Autodesk Inventor part; units mm, degrees
ref_plane "YZ Plane" through (0, 0, 0) normal (1, 0, 0) x (0, 1, 0)
ref_plane "XZ Plane" through (0, 0, 0) normal (0, 1, 0) x (-1, 0, 0)
ref_plane "XY Plane" through (0, 0, 0) normal (0, 0, 1) x (1, 0, 0)
sketch "スケッチ1" plane through (0, 0, 0) normal (0, 1, 0) x (-1, 0, 0)
  line L0 (37.5, 1.5) -> (-37.5, 1.5)
  line L1 (-37.5, 1.5) -> (-37.5, -1.5)
  line L2 (-37.5, -1.5) -> (37.5, -1.5)
  line L3 (37.5, -1.5) -> (37.5, 1.5)
  line L4 (37.5, 1.5) -> (-37.5, -1.5) construction
  line L5 (-37.5, 1.5) -> (37.5, -1.5) construction
  line L6 (36.5, 3.5) -> (38.5, 3.5)
  line L7 (38.5, 3.5) -> (38.5, -3.5)
  line L8 (38.5, -3.5) -> (36.5, -3.5)
  line L9 (36.5, -3.5) -> (36.5, 3.5)
  line L10 (36.5, 3.5) -> (38.5, -3.5) construction
  line L11 (38.5, 3.5) -> (36.5, -3.5) construction
  line L12 (-36.5, 3.5) -> (-38.5, 3.5)
  line L13 (-38.5, 3.5) -> (-38.5, -3.5)
  line L14 (-38.5, -3.5) -> (-36.5, -3.5)
  line L15 (-36.5, -3.5) -> (-36.5, 3.5)
  line L16 (-36.5, 3.5) -> (-38.5, -3.5) construction
  line L17 (-38.5, 3.5) -> (-36.5, -3.5) construction
  point P0 (0, 0)
  point P1 (37.5, 0)
  point P2 (-37.5, 0)
  dimension "d0" = 75
  dimension "d1" = 3
  dimension "d2" = 2
  dimension "d3" = 7
  dimension "d4" = 2
  dimension "d5" = 7
extrude "押し出し1" add sketch "スケッチ1" along normal blind 78
sketch "スケッチ2" plane through (0, 78, 0) normal (0, 1, 0) x (1, 0, 0)
  line L0 (1.55, -1.5) -> (-1.55, -1.5)
  line L1 (-1.55, -1.5) -> (-1.55, 1.5)
  line L2 (-1.55, 1.5) -> (1.55, 1.5)
  line L3 (1.55, 1.5) -> (1.55, -1.5)
  line L4 (1.55, -1.5) -> (-1.55, 1.5) construction
  line L5 (-1.55, -1.5) -> (1.55, 1.5) construction
  point P0 (0, 0)
  dimension "d8" = 3.1
  dimension "d9" = 3
extrude "押し出し2" cut sketch "スケッチ2" against normal blind 39
fillet "フィレット1" radius 0.5 33 edges at (19.025, 78, -1.5) (19.025, 78, 1.5) (1.55, 78, 0) (1.55, 58.5, 1.5) (1.55, 58.5, -1.5) (-1.55, 58.5, -1.5) (0, 39, -1.5) (0, 39, 1.5) (-1.55, 58.5, 1.5) (-1.55, 78, 0) (-19.025, 78, 1.5) (-19.025, 78, -1.5) (36.5, 78, 2.5) (37.5, 78, 3.5) (38.5, 78, 0) (37.5, 78, -3.5) (36.5, 78, -2.5) (36.5, 39, -3.5) (38.5, 39, -3.5) (38.5, 39, 3.5) (36.5, 39, 3.5) (-36.5, 39, 3.5) (-37.5, 78, 3.5) (-36.5, 78, 2.5) (-38.5, 78, 0) (-36.5, 78, -2.5) (-37.5, 78, -3.5) (-36.5, 39, -3.5) (-38.5, 39, -3.5) (-38.5, 39, 3.5) (-38.5, 0, 0) (-37.5, 0, 3.5) (-36.5, 0, 2.5)
fillet "フィレット2" radius 0.5 20 edges at (-36.75, 0, 1.5) (0, 0, 1.5) (0, 0, -1.5) (-37, 0, -2.25) (-37, 0, 2.25) (-37.5, 0, 3) (36.6464, 0, 3.3536) (-38, 0, 0) (-37.5, 0, -3) (38.3536, 0, 3.3536) (38.3536, 0, -3.3536) (36.6462, 0, -3.3538) (-38.3536, 0.1464, 3) (-38.5, 0.5, 0) (-38.3536, 0.1464, -3) (37.5, 0, 3.5) (38.5, 0, 0) (37.4995, 0, -3.5) (36.5, 0, -2.2505) (36.5, 0, 2.25)
properties part number "partition"
Source: CAD feature listing. Evaluate the final solid. Frame: model axes, mm. A direction names the side the tool comes from. Coordinates: 2 decimals unless noted, no trailing zeros. Loops run counter-clockwise (first coordinate to the right, second up) from the corner with the lowest first, then second, coordinate; pieces in that order, holes last. Notation, with made-up numbers: (86, 73.25) -> (125, 73.25) arc R10 cw to (125, 87.25) -> close; hole circle Ø1 at (41, -39.75). An arc over 180 degrees is marked (long way). One line per item, written item: value. Start each with the question number.
Q1. Section query C-C, the plane y = 20. Return the cut outline in (x, z), and give its area (3 significant figures).
Q2. Section query B-B, the plane x = -8.5. Return the cut outline in (y, z), and give its area (3 significant figures).
Q3. Section query A-A, the plane y = 63. Return the cut outline in (x, z), and give its area (3 significant figures).
Q4. Mould query, pull axis X, two halves, no side actions, for faces 1 (the face through (21, 78, 0)), 2 (the face through (1, 38, -1.5)), 3 (the face through (38.5, 38, 0)). Classes: pulls with the +X half, pulls with the -X half, needs draft (parallel to the pull), parting line crosses it, or undercut.
Q5. Set-up query: faces 4 (the face through (1.55, 59, 0)), 5 (the face through (-1, 38, 1.5)), 6 (the face through (-38.5, 38, 0)). Return all of +Z, -Z, +X, -X, +Y, -Y with unobstructed straight access to the full face (end or side cutting, diameter ignored); none if empty.
Q6. Contact query for flat-ended pins moving along their axis: P1, Ø1, axis at x = -22, y = 16, coming from the -Z side; P2, Ø1, axis at x = -15, y = 27.5, coming from the +Z side; P3, Ø1, axis at x = -0.5, z = 0, coming from the +Y side. Output: stop coordinate, or through.
Q7. Line query: line 1 along X through (y, z) = (57.5, 0); line 2 along X through (y, z) = (47, -2.75); line 3 along Z through (x, y) = (-34, 20.5). Output: solid intervals per line, ascending.
Results:
1. outline: (-38.5, -3) arc R0.5 ccw to (-38, -3.5) -> (-37, -3.5) arc R0.5 ccw to (-36.5, -3) -> (-36.5, -1.5) -> (36.5, -1.5) -> (36.5, -3) arc R0.5 ccw to (37, -3.5) -> (38, -3.5) arc R0.5 ccw to (38.5, -3) -> (38.5, 3) arc R0.5 ccw to (38, 3.5) -> (37, 3.5) arc R0.5 ccw to (36.5, 3) -> (36.5, 1.5) -> (-36.5, 1.5) -> (-36.5, 3) arc R0.5 ccw to (-37, 3.5) -> (-38, 3.5) arc R0.5 ccw to (-38.5, 3) -> close
1. area: 247 mm^2
2. outline: (0, -1) arc R0.5 ccw to (0.5, -1.5) -> (77.5, -1.5) arc R0.5 ccw to (78, -1) -> (78, 1) arc R0.5 ccw to (77.5, 1.5) -> (0.5, 1.5) arc R0.5 ccw to (0, 1) -> close
2. area: 234 mm^2
3. outline: (-38.5, -3) arc R0.5 ccw to (-38, -3.5) -> (-37, -3.5) arc R0.5 ccw to (-36.5, -3) -> (-36.5, -1.5) -> (-2.05, -1.5) arc R0.5 ccw to (-1.55, -1) -> (-1.55, 1) arc R0.5 ccw to (-2.05, 1.5) -> (-36.5, 1.5) -> (-36.5, 3) arc R0.5 ccw to (-37, 3.5) -> (-38, 3.5) arc R0.5 ccw to (-38.5, 3) -> close; (1.55, -1) arc R0.5 ccw to (2.05, -1.5) -> (36.5, -1.5) -> (36.5, -3) arc R0.5 ccw to (37, -3.5) -> (38, -3.5) arc R0.5 ccw to (38.5, -3) -> (38.5, 3) arc R0.5 ccw to (38, 3.5) -> (37, 3.5) arc R0.5 ccw to (36.5, 3) -> (36.5, 1.5) -> (2.05, 1.5) arc R0.5 ccw to (1.55, 1) -> close
3. area: 237 mm^2
4. face 1: needs draft
4. face 2: undercut
4. face 3: pulls with the +X half
5. face 4: +Z, -Z, +Y
5. face 5: +Z, +Y, -Y
5. face 6: +Z, -Z, -X, +Y, -Y
6. P1: z = -1.5
6. P2: z = 1.5
6. P3: y = 39
7. line 1: -38.5 to -1.55, 1.55 to 38.5
7. line 2: -38.5 to -36.5, 36.5 to 38.5
7. line 3: -1.5 to 1.5
